Source: CAD feature listing. Evaluate the final solid. Frame: model axes, mm. A direction names the side the tool comes from. Round coordinates to 2 decimals unless told otherwise and drop trailing zeros. Loops run counter-clockwise (first coordinate to the right, second up) from the corner with the lowest first, then second, coordinate; pieces in that order, holes last. Notation, with made-up numbers: (-12, 2) - (40, 2) arc R19 ccw to (40, 12) - close; hole circle Ø10 at (45, -38.75). An arc over 180 degrees is marked (long way). One line per question, with ' | ' between items. Start each with the question number.
1. Access query for faces 4 (the flat face through (436, -21, 47)), 5 (the flat face through (221, -43.7, 47)). Directions: +Z, -Z, +X, -X, +Y, -Y. A direction counts if a zero-diameter tool reaches every point of the face in a straight line with its end or side. Return the directions, or none.
2. Cut plane C-C (z = 56). Return loops of the section in (x, y), then the cut area to 3 significant figures.
3. Ray query, line 1 (X direction, y = -22.5, z = 84); line 2 (Y direction, x = 321, z = 77); line 3 (X direction, y = -44, z = 70). Return the intervals inside material, ascending.
4. Pin query (flat end, axial travel): pin 1 (1.5 mm diameter, centred on x = 154.5, z = 50, fed in from +Y); pin 2 (2 mm diameter, centred on y = -5, z = 75, fed in from -X). Return the tip coordinate at first contact, or that it passes through.
5. Cut plane A-A (y = -33.5). Return loops of the section in (x, z), then the cut area to 3 significant figures.
6. Mould query, pull axis X, two halves, no side actions, for faces 1 (the flat face through (0, -21, 47)), 2 (the flat face through (2, -21, 47)), 3 (the flat face through (217, -45, 96)). Classes: pulls with the +X half, pulls with the -X half, needs draft (parallel to the pull), parting line crosses it, or undercut.
7. Cut plane B-B (z = 76). Return loops of the section in (x, y).
8. Cut plane D-D (x = 62.5). Return loops of the section in (y, z), then the cut area to 3 significant figures.
```python
from build123d import *

# Parameters (mm, degrees)
SM_BASE_FLANGE_1_DEPTH = 96
SKETCH_2_R             = 2.3
CUT_EXTRUDE_1_DEPTH    = 449.776659375
CHAMFER_1_SIZE         = 2.05


# Sheet-metal steps are written as plain solids
with BuildPart() as part:
    # Sketch 1 → Базовая кромка1 (new body)
    with BuildSketch(Plane.XY):
        with BuildLine():
            Line((0, 0), (0, -41.7))
            ThreePointArc((0, -41.7), (1.171572875, -44.528427125), (4, -45.7))
            Line((4, -45.7), (432, -45.7))
            ThreePointArc((432, -45.7), (434.828427125, -44.528427125), (436, -41.7))
            Line((436, -41.7), (436, 0))
            Line((436, 0), (434, 0))
            Line((434, 0), (434, -41.7))
            ThreePointArc((434, -41.7), (433.414213562, -43.114213562), (432, -43.7))
            Line((432, -43.7), (4, -43.7))
            ThreePointArc((4, -43.7), (2.585786438, -43.114213562), (2, -41.7))
            Line((2, -41.7), (2, 0))
            Line((2, 0), (0, 0))
        make_face()
    extrude(amount=SM_BASE_FLANGE_1_DEPTH)

    # Sketch 2 → Вырез-Вытянуть1 (cut, through all)
    with BuildSketch(Plane.ZY):
        with Locations(Location((20, -8, 0), (0, 0, 270))):
            Circle(SKETCH_2_R)
        with Locations(Location((76, -8, 0), (0, 0, 270))):
            Circle(SKETCH_2_R)
    extrude(amount=-CUT_EXTRUDE_1_DEPTH, mode=Mode.SUBTRACT)

    # Фаска1
    # the kernel refuses this chamfer: 2.05 mm, written as the material it takes off along each edge
    with BuildSketch(Plane(origin=(436, -8, 20), x_dir=(0, -1, 0), z_dir=(0, 0, -1))) as chamfer_1_piece_1:
        Polygon((2.3 + CHAMFER_1_SIZE, 0), (2.3, CHAMFER_1_SIZE), (2.3, 0), align=None)
    revolve(axis=Axis((436, -8, 20), (-1, 0, 0)), mode=Mode.SUBTRACT)
    with BuildSketch(Plane(origin=(436, -8, 76), x_dir=(0, -1, 0), z_dir=(0, 0, -1))) as chamfer_1_piece_2:
        Polygon((2.3 + CHAMFER_1_SIZE, 0), (2.3, CHAMFER_1_SIZE), (2.3, 0), align=None)
    revolve(axis=Axis((436, -8, 76), (-1, 0, 0)), mode=Mode.SUBTRACT)
    with BuildSketch(Plane(origin=(0, -8, 76), x_dir=(0, -1, 0), z_dir=(0, 0, -1))) as chamfer_1_piece_3:
        Polygon((2.3, -CHAMFER_1_SIZE), (2.3 + CHAMFER_1_SIZE, 0), (2.3, 0), align=None)
    revolve(axis=Axis((0, -8, 76), (-1, 0, 0)), mode=Mode.SUBTRACT)
    with BuildSketch(Plane(origin=(0, -8, 20), x_dir=(0, -1, 0), z_dir=(0, 0, -1))) as chamfer_1_piece_4:
        Polygon((2.3, -CHAMFER_1_SIZE), (2.3 + CHAMFER_1_SIZE, 0), (2.3, 0), align=None)
    revolve(axis=Axis((0, -8, 20), (-1, 0, 0)), mode=Mode.SUBTRACT)


solid = part.part
```
Answers follow:
1) face 4: +Z, -Z, +X, +Y, -Y | face 5: +Z, -Z, +Y
2) outline: (0, -41.7) arc R4 ccw to (4, -45.7) - (432, -45.7) arc R4 ccw to (436, -41.7) - (436, 0) - (434, 0) - (434, -41.7) arc R2 cw to (432, -43.7) - (4, -43.7) arc R2 cw to (2, -41.7) - (2, 0) - (0, 0) - close | area: 1,040 mm2
3) line 1: x = 0 to 2, 434 to 436 | line 2: y = -45.7 to -43.7 | line 3: x = 0.73 to 435.27
4) pin 1: stops at y = -43.7 | pin 2: stops at x = 0.19
5) outline: (0, 0) - (2, 0) - (2, 96) - (0, 96) - close; (434, 0) - (436, 0) - (436, 96) - (434, 96) - close | area: 384 mm2
6) face 1: pulls with the -X half | face 2: undercut | face 3: needs draft
7) outline: (0, -41.7) arc R4 ccw to (4, -45.7) - (432, -45.7) arc R4 ccw to (436, -41.7) - (436, -12.35) - (434, -10.35) - (434, -41.7) arc R2 cw to (432, -43.7) - (4, -43.7) arc R2 cw to (2, -41.7) - (2, -10.35) - (0, -12.35) - close; (0, -3.65) - (2, -5.65) - (2, 0) - (0, 0) - close; (434, -5.65) - (436, -3.65) - (436, 0) - (434, 0) - close
8) outline: (-45.7, 0) - (-43.7, 0) - (-43.7, 96) - (-45.7, 96) - close | area: 192 mm2
